Autodesk Fusion 360 part; units mm, degrees
sketch "Sketch1" plane through (0, 0, 0) normal (0, 0, 1) x (1, 0, 0)
  line L0 (-15.6254, 36.106) -> (47.1246, 36.106)
  line L1 (47.1246, 36.106) -> (47.1246, -41.1843)
  line L2 (47.1246, -41.1843) -> (-15.6254, -41.1843)
  line L3 (-15.6254, -41.1843) -> (-15.6254, 36.106)
  line L4 (-25.6254, 46.106) -> (57.1246, 46.106)
  line L5 (57.1246, 46.106) -> (57.1246, -51.1843)
  line L6 (57.1246, -51.1843) -> (-25.6254, -51.1843)
  line L7 (-25.6254, -51.1843) -> (-25.6254, 46.106)
  circle A0 centre (-20.6254, 41.106) radius 1.45
  circle A1 centre (52.5, 41.106) radius 1.45
  circle A2 centre (52.1246, -46.1843) radius 1.45
  circle A3 centre (-20.6254, -46.1843) radius 1.45
  dimension "d1" = 77.2903
  dimension "d2" = 62.75
  dimension "d3" = 10
  dimension "d4" = 10
  dimension "d5" = 10
  dimension "d6" = 10
  dimension "d7" = 2.9
  dimension "d8" = 5
  dimension "d9" = 5
  dimension "d10" = 2.9
  dimension "d11" = 2.9
  dimension "d12" = 2.9
  dimension "d13" = 5
  dimension "d14" = 5
  dimension "d15" = 5
  dimension "d16" = 5
  dimension "d17" = 5
extrude "Extrude3" add sketch "Sketch1" along normal blind 3 contours L0 L1 L2 L3
extrude "Extrude4" add sketch "Sketch1" along normal blind 13
sketch "Sketch3" plane through (0, -51.1843, 0) normal (0, -1, 0) x (1, 0, 0)
  line L0 (-25.6254, 0) -> (57.1246, 0)
  line L1 (57.1246, 0) -> (57.1246, 13)
  line L2 (57.1246, 13) -> (-25.6254, 13)
  line L3 (-25.6254, 13) -> (-25.6254, 0)
  line L4 (17.2996, 13) -> (35.7996, 13)
  line L5 (35.7996, 13) -> (35.7996, 3)
  line L6 (35.7996, 3) -> (17.2996, 3)
  line L7 (17.2996, 3) -> (17.2996, 13)
  dimension "d26" = 21.325
  dimension "d27" = 18.5
extrude "Extrude5" cut sketch "Sketch3" against normal blind 13 contours L2 L4 L5 L6 L7
fillet "Fillet1" radius 5 4 edges at (57.1246, 46.106, 6.5) (-25.6254, 46.106, 6.5) (-25.6254, -51.1843, 6.5) (57.1246, -51.1843, 6.5)
extrude "Extrude1" [suppressed]
extrude "Extrude2" [suppressed]
The model under review builds one solid part; all positions refer to its coordinate system, in mm. A direction names the side the tool comes from. Round coordinates to 2 decimals unless told otherwise and drop trailing zeros. Write each loop counter-clockwise with the first axis right and the second up, starting at its lowest first coordinate (ties: lowest second). Pieces come first, ordered by that corner, then holes. Notation, with made-up numbers: (46.25, -34) -> (72.25, -34) arc R23 cw to (72.25, -22) -> close; hole circle Ø11 at (-27, 20). An arc over 180 degrees is marked (long way). Answer as a JSON object with one key per item and string values.
1. Machinability: for faces 1 (the face through (1, -41.184, 8)), 2 (the face through (-19.956, 42.392, 6.409)), 3 (the face through (17.3, -46, 8)), which of the approach directions +Z, -Z, +X, -X, +Y, -Y give a long, thin tool a straight path to every point of the face, cutting with its end or side? Answer none if there is none.
Results found:
{"face 1": "+Z", "face 2": "+Z, -Z", "face 3": "+Z, -Y"}
2. We need section C-C on x = 10. State the section outline as (y, z) points, and give its area (3 significant figures).
Results found:
{"outline": "(-51.18, 0) -> (46.11, 0) -> (46.11, 13) -> (36.11, 13) -> (36.11, 3) -> (-41.18, 3) -> (-41.18, 13) -> (-51.18, 13) -> close", "area": "492 mm^2"}
3. To check wall thickness, follow line 1 along Y through (x, z) = (-1.5, 4.5); line 2 along X through (y, z) = (41, 4.75); line 3 along X through (y, z) = (-43.5, 9.25). State the ranges of each line that lie inside material, in increasing order.
Results found:
{"line 1": "y = -51.18 to -41.18, 36.11 to 46.11", "line 2": "x = -25.63 to -22.07, -19.18 to 51.05, 53.95 to 57.12", "line 3": "x = -25.63 to 17.3, 35.8 to 57.12"}
4. We need section B-B on y = -9. State the section outline as (x, z) points.
Results found:
{"outline": "(-25.63, 0) -> (57.12, 0) -> (57.12, 13) -> (47.12, 13) -> (47.12, 3) -> (-15.63, 3) -> (-15.63, 13) -> (-25.63, 13) -> close"}
5. The part is to be moulded in two halves that separate along X. For faces 4 (the face through (55.62, -49.76, 6.59)), 5 (the face through (35.8, -46, 8)), 6 (the face through (-18, 1, 13)), 7 (the face through (-24.1, 44.7, 6.6)), say which applies: pulls with the +X half, pulls with the -X half, needs draft (parallel to the pull), parting line crosses it, or undercut.
Results found:
{"face 4": "pulls with the +X half", "face 5": "undercut", "face 6": "needs draft", "face 7": "pulls with the -X half"}
6. We need section A-A on z = 7.5. State the section outline as (x, y) points, and give its area (3 significant figures).
Results found:
{"outline": "(-25.63, -46.18) arc R5 ccw to (-20.63, -51.18) -> (17.3, -51.18) -> (17.3, -41.18) -> (-15.63, -41.18) -> (-15.63, 36.11) -> (47.12, 36.11) -> (47.12, -41.18) -> (35.8, -41.18) -> (35.8, -51.18) -> (52.12, -51.18) arc R5 ccw to (57.12, -46.18) -> (57.12, 41.11) arc R5 ccw to (52.12, 46.11) -> (-20.63, 46.11) arc R5 ccw to (-25.63, 41.11) -> close; hole circle Ø2.9 at (-20.63, -46.18); hole circle Ø2.9 at (-20.63, 41.11); hole circle Ø2.9 at (52.12, -46.18); hole circle Ø2.9 at (52.5, 41.11)", "area": "2,970 mm^2"}
7. Clearance check with flat-ended pins moving along their axes: pin 1 (3 mm diameter, centred on x = -12.5, y = -23, fed in from -Z); pin 2 (2.5 mm diameter, centred on x = 52.12, y = -46.18, fed in from -Z); pin 3 (19 mm diameter, centred on x = 27.5, y = -3, fed in from +Z). State where each tip first meets the part, or that it passes through.
Results found:
{"pin 1": "stops at z = 0", "pin 2": "passes through", "pin 3": "stops at z = 3"}
